CAD build for the part. Positions are in the model's coordinates, mm. Face numbers are marked on the shaded views. Coordinates: 2 decimals unless noted, no trailing zeros. Loops run counter-clockwise (first coordinate to the right, second up) from the corner with the lowest first, then second, coordinate; pieces in that order, holes last. Notation, with made-up numbers: (-16, 59) -> (-3, 59) arc R21 ccw to (-3, 83) -> close; hole circle Ø11 at (59.5, 15). An arc over 180 degrees is marked (long way). Answer as a JSON object with one key per item and string values. Group by question number.
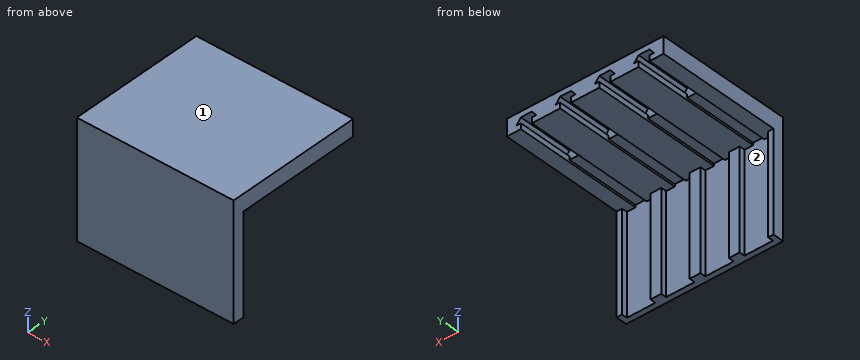
from build123d import *

# Parameters (mm, degrees)
SKETCH1_W               = 35.5
SKETCH1_H               = 105
BOSS_EXTRUDE1_DEPTH     = 10
SKETCH2_W               = 35.5
SKETCH2_H               = 15
BOSS_EXTRUDE2_DEPTH     = 113
SKETCH5_W               = 25.7
SKETCH5_H               = 90
CUT_EXTRUDE2_DEPTH      = 5
CUT_EXTRUDE3_DEPTH      = 50
SKETCH7_W               = 10
SKETCH7_H               = 2
CUT_EXTRUDE4_DEPTH      = 68
LPATTERN1_DEPTH         = 123
LPATTERN1_2_DEPTH       = 5
LPATTERN1_START         = 5
LPATTERN1_3_DEPTH       = 68
LPATTERN1_4_OUTLINE_W   = 9.8
LPATTERN1_4_OUTLINE_H   = 90
LPATTERN1_4_OUTLINE_W_2 = 4.9
LPATTERN1_4_DEPTH       = 5


# Read off the part's stored shape, not the designer's step: LPattern1
with BuildPart() as part:
    # Sketch1 → Boss-Extrude1 (new body)
    with BuildSketch(Plane(origin=(0, 0, 0), x_dir=(1, 0, 0), z_dir=(0, 1, 0))):
        Rectangle(SKETCH1_W, SKETCH1_H)
    extrude(amount=BOSS_EXTRUDE1_DEPTH)

    # Sketch2 → Boss-Extrude2 (add)
    with BuildSketch(Plane(origin=(0, 10, 0), x_dir=(1, 0, 0), z_dir=(0, 1, 0))):
        with Locations((0, -45)):
            Rectangle(SKETCH2_W, SKETCH2_H)
    extrude(amount=BOSS_EXTRUDE2_DEPTH)

    # Sketch5 → Cut-Extrude2 (cut)
    with BuildSketch(Plane(origin=(0, 10, 0), x_dir=(1, 0, 0), z_dir=(0, 1, 0))):
        with Locations((0, 7.5)):
            Rectangle(SKETCH5_W, SKETCH5_H)
    extrude(amount=-CUT_EXTRUDE2_DEPTH, mode=Mode.SUBTRACT)

    # Sketch6 → Cut-Extrude3 (cut)
    with BuildSketch(Plane(origin=(0, 123, 0), x_dir=(1, 0, 0), z_dir=(0, 1, 0))):
        Polygon((-5, -37.5), (5, -37.5), (5, -42.5), (9, -42.5), (5, -47.5), (-5, -47.5), (-9, -42.5), (-5, -42.5), align=None)
    extrude(amount=-CUT_EXTRUDE3_DEPTH, mode=Mode.SUBTRACT)

    # Sketch7 → Cut-Extrude4 (cut)
    with BuildSketch(Plane(origin=(0, 73, 0), x_dir=(1, 0, 0), z_dir=(0, 1, 0))):
        with Locations((0, -38.5)):
            Rectangle(SKETCH7_W, SKETCH7_H)
    extrude(amount=-CUT_EXTRUDE4_DEPTH, mode=Mode.SUBTRACT)

    # LPattern1 outline → LPattern1 (add)
    with BuildSketch(Plane(origin=(0, 0, 0), x_dir=(1, 0, 0), z_dir=(0, 1, 0))):
        Polygon((-40.5, -37.5), (-66, -37.5), (-66, -42.5), (-62, -42.5), (-66, -47.5), (-76, -47.5), (-80, -42.5), (-76, -42.5), (-76, -37.5), (-101.5, -37.5), (-101.5, -42.5), (-97.5, -42.5), (-101.5, -47.5), (-111.5, -47.5), (-115.5, -42.5), (-111.5, -42.5), (-111.5, -37.5), (-124.25, -37.5), (-124.25, -52.5), (-17.75, -52.5), (-17.75, -37.5), (-30.5, -37.5), (-30.5, -42.5), (-26.5, -42.5), (-30.5, -47.5), (-40.5, -47.5), (-44.5, -42.5), (-40.5, -42.5), align=None)
    extrude(amount=LPATTERN1_DEPTH)

    # LPattern1 2 outline → LPattern1 2 (add)
    with BuildSketch(Plane(origin=(0, 0, 0), x_dir=(1, 0, 0), z_dir=(0, 1, 0))):
        Polygon((-66, -37.5), (-40.5, -37.5), (-40.5, -42.5), (-44.5, -42.5), (-40.5, -47.5), (-30.5, -47.5), (-26.5, -42.5), (-30.5, -42.5), (-30.5, -37.5), (-17.75, -37.5), (-17.75, 52.5), (-124.25, 52.5), (-124.25, -37.5), (-111.5, -37.5), (-111.5, -42.5), (-115.5, -42.5), (-111.5, -47.5), (-101.5, -47.5), (-97.5, -42.5), (-101.5, -42.5), (-101.5, -37.5), (-76, -37.5), (-76, -42.5), (-80, -42.5), (-76, -47.5), (-66, -47.5), (-62, -42.5), (-66, -42.5), align=None)
    extrude(amount=LPATTERN1_2_DEPTH)

    # LPattern1 3 outline → LPattern1 3 (add)
    with BuildSketch(Plane(origin=(0, 0, 0), x_dir=(1, 0, 0), z_dir=(0, 1, 0)).offset(LPATTERN1_START)):
        Polygon((-66, -42.5), (-66, -39.5), (-76, -39.5), (-76, -42.5), (-80, -42.5), (-76, -47.5), (-66, -47.5), (-62, -42.5), align=None)
        Polygon((-30.5, -39.5), (-40.5, -39.5), (-40.5, -42.5), (-44.5, -42.5), (-40.5, -47.5), (-30.5, -47.5), (-26.5, -42.5), (-30.5, -42.5), align=None)
        Polygon((-101.5, -42.5), (-101.5, -39.5), (-111.5, -39.5), (-111.5, -42.5), (-115.5, -42.5), (-111.5, -47.5), (-101.5, -47.5), (-97.5, -42.5), align=None)
    extrude(amount=LPATTERN1_3_DEPTH)

    # LPattern1 4 outline → LPattern1 4 (add)
    with BuildSketch(Plane(origin=(0, 0, 0), x_dir=(1, 0, 0), z_dir=(0, 1, 0)).offset(LPATTERN1_START)):
        with Locations((-53.25, 7.5)):
            Rectangle(LPATTERN1_4_OUTLINE_W, LPATTERN1_4_OUTLINE_H)
        with Locations((-88.75, 7.5)):
            Rectangle(LPATTERN1_4_OUTLINE_W, LPATTERN1_4_OUTLINE_H)
        with Locations((-20.2, 7.5)):
            Rectangle(LPATTERN1_4_OUTLINE_W_2, LPATTERN1_4_OUTLINE_H)
        with Locations((-121.8, 7.5)):
            Rectangle(LPATTERN1_4_OUTLINE_W_2, LPATTERN1_4_OUTLINE_H)
    extrude(amount=LPATTERN1_4_DEPTH)


solid = part.part
Item 1: Band-saw the part on B-B, the plane x = 1.5. List the corners of the cut face in (y, z).
Item 2: Band-saw the part on C-C, the plane z = -43.5. List the corners of the cut face in (x, y).
Item 3: Pull direction X, two halves, no side cores. Call the marked faces 1 and 2: +X half, -X half, draft (parallel to the pull), parting line (faces both ways), or undercut.
Item 4: Drill centre lines: L1, parallel to Y at x = -34.5, z = -24; L2, parallel to Y at x = -107, z = 44; L3, parallel to Z at x = -23.5, y = 60. Where is each one in solid material? Low to high.
Item 5: Flat gauge pins, fed straight in: P1, Ø5, axis at x = -55.5, y = 15.5, coming from the -Z side; P2, Ø3, axis at x = -33.5, y = 95.5, coming from the -Z side; P3, Ø3, axis at x = -55.5, z = -5.5, coming from the +Y side. Where does each tip first touch, or does it go through?
Item 6: Band-saw the part on A-A, the plane y = 31. List the corners of the cut face in (x, z), and give its area (3 significant figures).
Item 7: Band-saw the part on D-D, the plane x = -89. List the corners of the cut face in (y, z).
Reply:
{
 "1": {"outline": "(0, -52.5) -> (5, -52.5) -> (5, 39.5) -> (73, 39.5) -> (73, 47.5) -> (123, 47.5) -> (123, 52.5) -> (0, 52.5) -> close"},
 "2": {"outline": "(-124.25, 0) -> (17.75, 0) -> (17.75, 10) -> (12.85, 10) -> (12.85, 5) -> (-12.85, 5) -> (-12.85, 10) -> (-22.65, 10) -> (-22.65, 5) -> (-48.35, 5) -> (-48.35, 10) -> (-58.15, 10) -> (-58.15, 5) -> (-83.85, 5) -> (-83.85, 10) -> (-93.65, 10) -> (-93.65, 5) -> (-119.35, 5) -> (-119.35, 10) -> (-124.25, 10) -> close"},
 "3": {"face 1": "draft", "face 2": "undercut"},
 "4": {"L1": "0 to 5", "L2": "0 to 73", "L3": "37.5 to 52.5"},
 "5": {"P1": "z = 37.5", "P2": "z = 47.5", "P3": "y = 10"},
 "6": {"outline": "(-124.25, 37.5) -> (-111.5, 37.5) -> (-111.5, 39.5) -> (-101.5, 39.5) -> (-101.5, 37.5) -> (-76, 37.5) -> (-76, 39.5) -> (-66, 39.5) -> (-66, 37.5) -> (-40.5, 37.5) -> (-40.5, 39.5) -> (-30.5, 39.5) -> (-30.5, 37.5) -> (-5, 37.5) -> (-5, 39.5) -> (5, 39.5) -> (5, 37.5) -> (17.75, 37.5) -> (17.75, 52.5) -> (-124.25, 52.5) -> close", "area": "2,050 mm²"},
 "7": {"outline": "(0, -52.5) -> (10, -52.5) -> (10, 37.5) -> (123, 37.5) -> (123, 52.5) -> (0, 52.5) -> close"}
}
